```python
from build123d import *

# Parameters (mm, degrees)
BOSS_EXTRUDE1_DEPTH = 80
SKETCH2_W           = 80
SKETCH2_H           = 10
BOSS_EXTRUDE2_DEPTH = 25


with BuildPart() as part:
    # Sketch1 → Boss-Extrude1 (new body)
    with BuildSketch(Plane(origin=(0, 0, 0), x_dir=(1, 0, 0), z_dir=(0, 1, 0))):
        Polygon((-60, 0), (60, 0), (80, -15), (83, -11), (61.666666667, 5), (-61.666666667, 5), (-83, -11), (-80, -15), align=None)
    extrude(amount=-BOSS_EXTRUDE1_DEPTH)

    # Sketch2 → Boss-Extrude2 (add)
    with BuildSketch(Plane(origin=(0, 0, -5), x_dir=(-1, 0, 0), z_dir=(0, 0, -1))):
        with Locations((0, -60)):
            Rectangle(SKETCH2_W, SKETCH2_H)
    extrude(amount=BOSS_EXTRUDE2_DEPTH)


solid = part.part
```
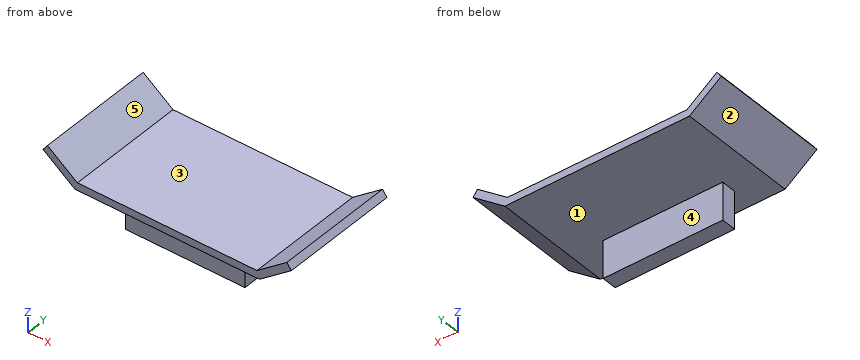
Here's how the part is built. I have some questions about the finished solid (model axes, mm). Face numbers are marked on the shaded views. A direction names the side the tool comes from. Coordinates: 2 decimals unless noted, no trailing zeros. Write each loop counter-clockwise with the first axis right and the second up, starting at its lowest first coordinate (ties: lowest second). Pieces come first, ordered by that corner, then holes. Notation, with made-up numbers: (88.5, -3.75) -> (123.5, -3.75) arc R16 cw to (123.5, 23.25) -> close; hole circle Ø9 at (-35.75, -37.75). An arc over 180 degrees is marked (long way). Use a Markdown table: item, result. Add a question column.
(1) Please list where these lines run through material, in increasing order: line 1 (Z direction, x = 52.5, y = -16); line 2 (X direction, y = -42.5, z = 7); line 3 (X direction, y = -43.5, z = 12).
(2) I'm going to push flat-ended pins straight in: P1, Ø10, axis at x = 58.5, y = -13, coming from the -Z side; P2, Ø3, axis at y = -61.5, z = -21, coming from the +X side; P3, Ø4, axis at x = 26.5, z = -20.5, coming from the -Y side; P4, Ø4, axis at x = 64.5, z = -1, coming from the +Y side. Where does each tip first touch, or does it pass through?
(3) If we section it at D-D, the plane z = -12.5: Write out the boundary of the cut face in (x, y).
(4) We'd pull the mould along X, two halves only. Please class the marked faces 1, 2 and 3: +X half, -X half, draft (parallel to the pull), parting line (faces both ways), or undercut.
(5) If we section it at C-C, the plane x = -20.5: Write out the boundary of the cut face in (y, z), and give its area (3 significant figures).
(6) If we section it at A-A, the plane z = 3.5: Write out the boundary of the cut face in (x, y), and give its area (3 significant figures).
(7) For the marked faces 4 and 5, which set-ups out of +Z, -Z, +X, -X, +Y, -Y let a thin tool reach every point of the face, with its end or its side?
(8) If we section it at B-B, the plane y = -31.5: Write out the boundary of the cut face in (x, z), and give its area (3 significant figures).
Outcome:
| question | item | result |
|---|---|---|
| 1 | line 1 | z = -5 to 0 |
| 1 | line 2 | x = -77.67 to -69.33, 69.33 to 77.67 |
| 1 | line 3 | x = -82.25 to -76, 76 to 82.25 |
| 2 | P1 | stops at z = -5 |
| 2 | P2 | stops at x = 40 |
| 2 | P3 | stops at y = -65 |
| 2 | P4 | stops at y = 0 |
| 3 | outline | (-40, -65) -> (40, -65) -> (40, -55) -> (-40, -55) -> close |
| 4 | face 1 | draft |
| 4 | face 2 | -X half |
| 4 | face 3 | undercut |
| 5 | outline | (-80, -5) -> (-65, -5) -> (-65, -30) -> (-55, -30) -> (-55, -5) -> (0, -5) -> (0, 0) -> (-80, 0) -> close |
| 5 | area | 650 mm^2 |
| 6 | outline | (-73, -80) -> (-64.67, -80) -> (-64.67, 0) -> (-73, 0) -> close; (64.67, -80) -> (73, -80) -> (73, 0) -> (64.67, 0) -> close |
| 6 | area | 1,330 mm^2 |
| 7 | face 4 | -Z, +X, -X, +Y |
| 7 | face 5 | +Z, +Y, -Y |
| 8 | outline | (-83, 11) -> (-61.67, -5) -> (61.67, -5) -> (83, 11) -> (80, 15) -> (60, 0) -> (-60, 0) -> (-80, 15) -> close |
| 8 | area | 867 mm^2 |
